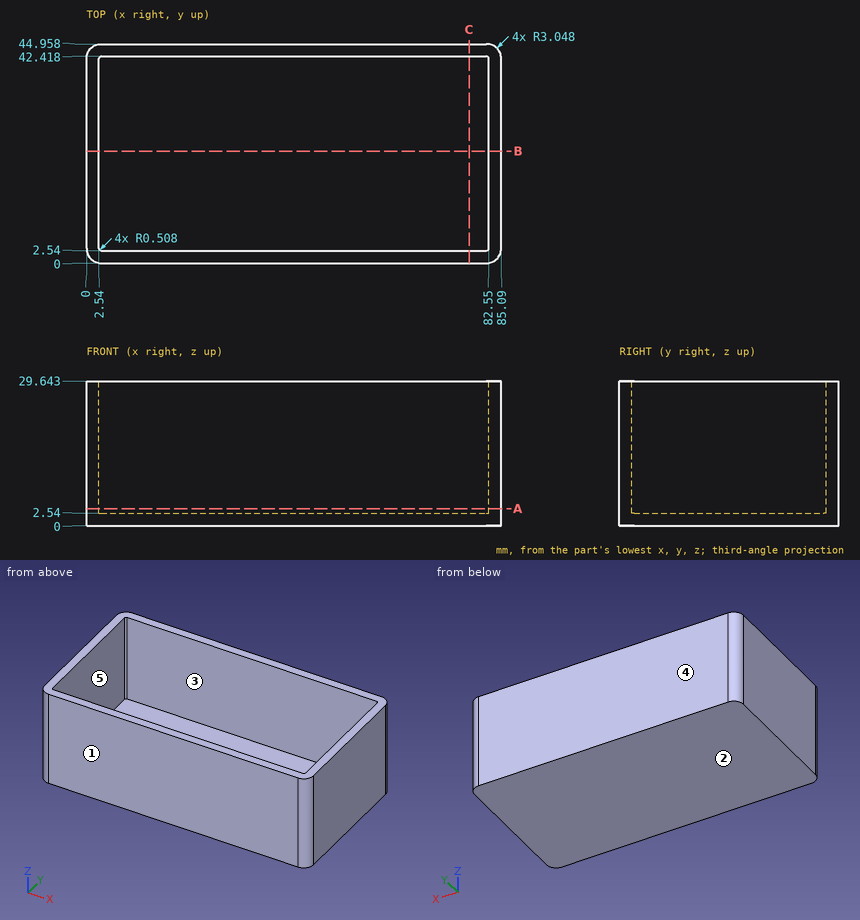
Geometry: see drawing. Coordinates: mm, zero at the bounding-box minimum. A direction names the side the tool comes from. Coordinates: 2 decimals unless noted, no trailing zeros. Loops run counter-clockwise (first coordinate to the right, second up) from the corner with the lowest first, then second, coordinate; pieces in that order, holes last. Notation, with made-up numbers: M 58,50 L 108,50 A19 ccw 108,59 Z; hole C -35.5,56.25 d2. An arc over 180 degrees is marked long. Put each result on its own line as item: value. Start each with the question number.
1) Ray query, L1, parallel to Y at x = 10, z = 24.75; L2, parallel to X at y = 8, z = 23.25; L3, parallel to Z at x = 13.5, y = 3.5. Return the intervals inside material, ascending. Write a range as from..to.
2) Cut plane B-B on y = 23. Return the cut outline in (x, z), then the cut area to 3 significant figures.
3) Cut plane C-C on x = 78.5. Return the cut outline in (y, z).
4) Cut plane A-A on z = 3.5. Return the cut outline in (x, y), then the cut area to 3 significant figures.
5) Contact query for a flat-ended pin moving along its axis: pin 1 Ø4 at (x, y) = (37, 34.5) entering from +Z. Output: stop coordinate, or through.
6) Pull-direction query (Y, two-part tool) for the marked faces 1, 2 and 3; classes: pulls with the +Y half, pulls with the -Y half, needs draft (parallel to the pull), parting line crosses it, or undercut.
7) Reachability of the marked faces 4 and 5 from +Z, -Z, +X, -X, +Y, -Y: full face, straight path, thin tool, end or side. Return the list, or none.
The answers:
1. L1: y = 0..2.54, 42.42..44.96
1. L2: x = 0..2.54, 82.55..85.09
1. L3: z = 0..2.54
2. outline: M 0,0 L 85.09,0 L 85.09,29.64 L 82.55,29.64 L 82.55,2.54 L 2.54,2.54 L 2.54,29.64 L 0,29.64 Z
2. area: 354 mm²
3. outline: M 0,0 L 44.96,0 L 44.96,29.64 L 42.42,29.64 L 42.42,2.54 L 2.54,2.54 L 2.54,29.64 L 0,29.64 Z
4. outline: M 0,3.05 A3.05 ccw 3.05,0 L 82.04,0 A3.05 ccw 85.09,3.05 L 85.09,41.91 A3.05 ccw 82.04,44.96 L 3.05,44.96 A3.05 ccw 0,41.91 Z; hole M 2.54,3.05 A0.51 ccw 3.05,2.54 L 82.04,2.54 A0.51 ccw 82.55,3.05 L 82.55,41.91 A0.51 ccw 82.04,42.42 L 3.05,42.42 A0.51 ccw 2.54,41.91 Z
4. area: 627 mm²
5. pin 1: stops at z = 2.54
6. face 1: pulls with the -Y half
6. face 2: needs draft
6. face 3: undercut
7. face 4: +Z, -Z, +X, -X, +Y
7. face 5: +Z
